Autodesk Inventor part; units mm, degrees
ref_plane "YZ Plane" through (0, 0, 0) normal (1, 0, 0) x (0, 1, 0)
ref_plane "XZ Plane" through (0, 0, 0) normal (0, 1, 0) x (-1, 0, 0)
ref_plane "XY Plane" through (0, 0, 0) normal (0, 0, 1) x (1, 0, 0)
sketch "Sketch1" plane through (0, 0, 0) normal (0, 1, 0) x (-1, 0, 0)
  line L0 (0, 0) -> (25, 0)
  line L1 (25, 0) -> (25, -10)
  line L2 (25, -10) -> (0, -10)
  line L3 (0, -10) -> (0, 0)
  dimension "d0" = 25
  dimension "d1" = 10
extrude "Extrusion1" add sketch "Sketch1" along normal blind 5
sketch "Sketch2" plane through (0, 5, 0) normal (0, 1, 0) x (1, 0, 0)
  line L0 (-25, 10) -> (-25, 0)
  line L1 (-25, 0) -> (0, 0)
  line L2 (-25, 10) -> (-20, 10)
  line L3 (-20, 10) -> (-20, 0)
  line L4 (-20, 0) -> (-25, 0)
  line L5 (-25, 0) -> (-25, 10)
  dimension "d4" = 5
extrude "Extrusion2" add sketch "Sketch2" along normal blind 45
sketch "Sketch3" plane through (0, 0, -10) normal (0, 0, -1) x (-1, 0, 0)
  point P0 (0, 0)
sketch "Sketch4" plane through (0, 0, -10) normal (0, 0, -1) x (-1, 0, 0)
  line L0 (0, 5) -> (20, 5)
  line L1 (0, 0) -> (0, 5)
  line L2 (0, 5) -> (0, 0)
  line L3 (0, 0) -> (25, 0)
  line L4 (25, 0) -> (25, 50)
  line L5 (25, 0) -> (25, 50)
  line L6 (20, 50) -> (25, 50)
  line L7 (25, 50) -> (20, 50)
  line L8 (20, 5) -> (20, 50)
  line L9 (20, 50) -> (20, 5)
  line L10 (20, 5) -> (0, 5)
extrude "Extrusion3" add sketch "Sketch4" along normal blind 14
Read the model definition and answer for the solid it produces. Units are mm, in the model's axes. A direction names the side the tool comes from. Give positions to 0.01 mm unless a question says otherwise; leave off trailing zeros. Write each loop counter-clockwise with the first axis right and the second up, starting at its lowest first coordinate (ties: lowest second). Pieces come first, ordered by that corner, then holes. Notation, with made-up numbers: M -34.75,24.25 L -3.75,24.25 A33 cw -3.75,58.25 Z; hole C 10,75.5 d3. An arc over 180 degrees is marked long. One line per item, written item: value. Start each with the question number.
(1) Flat-ended cylindrical pins translate along their axes: pin 1 Ø12 at (y, z) = (19.5, -12) entering from +X; pin 2 Ø1.5 at (x, z) = (-19, -20) entering from +Y. Find the tip coordinate at first contact, or state that the pin passes through.
(2) Find the intervals of material crossed by line 1 (X direction, y = 40, z = -12.25); line 2 (Y direction, x = -3.75, z = -18.25), in increasing order.
(3) Find section C-C (y = 25). Determine the outline of the cut face in (x, z), plus the area to 3 significant figures.
(4) Find section A-A (z = -6). Determine the outline of the cut face in (x, y).
(5) Find section B-B (x = -16.75). Determine the outline of the cut face in (y, z), plus the area to 3 significant figures.
(6) A tool of negligible diameter and unlimited length cuts with its end or side. For faces 1 (the flat face through (-21, 17, 0)), 2 (the flat face through (-20, 27, -12)), from which of +Z, -Z, +X, -X, +Y, -Y can it reach the whole face along a straight path? Write none if from no direction.
Results below:
1. pin 1: stops at x = -20
1. pin 2: stops at y = 5
2. line 1: x = -25 to -20
2. line 2: y = 0 to 5
3. outline: M -25,-24 L -20,-24 L -20,0 L -25,0 Z
3. area: 120 mm^2
4. outline: M -25,0 L 0,0 L 0,5 L -20,5 L -20,50 L -25,50 Z
5. outline: M 0,-24 L 5,-24 L 5,0 L 0,0 Z
5. area: 120 mm^2
6. face 1: +Z, +X, -X, +Y, -Y
6. face 2: +Z, -Z, +X, +Y
